Autodesk Inventor part; units mm, degrees
ref_plane "YZ Plane" through (0, 0, 0) normal (1, 0, 0) x (0, 1, 0)
ref_plane "XZ Plane" through (0, 0, 0) normal (0, 1, 0) x (-1, 0, 0)
ref_plane "XY Plane" through (0, 0, 0) normal (0, 0, 1) x (1, 0, 0)
sketch "Sketch1" plane through (0, 0, 0) normal (0, 1, 0) x (-1, 0, 0)
  point P0 (0, 0)
sketch "Sketch2" plane through (0, 0, 0) normal (0, 1, 0) x (-1, 0, 0)
  line L0 (70, -12) -> (70, -66)
  line L1 (70, -66) -> (2, -66)
  line L2 (70, -12) -> (2, -12)
  line L3 (2, -66) -> (2, -12)
  point P0 (0, 0)
  point P1 (2, 0)
  dimension "d151" = 68
  dimension "d152" = 54
extrude "Extrusion1" add sketch "Sketch2" along normal blind 14
sketch "Sketch3" plane through (0, 14, 0) normal (0, 1, 0) x (1, 0, 0)
  point P0 (0, 0)
sketch "Sketch4" plane through (0, 14, 0) normal (0, 1, 0) x (1, 0, 0)
  line L0 (-2, 66) -> (-70, 66)
  line L1 (-30.4814, 66) -> (-28.4814, 66)
  line L2 (-28.4814, 66) -> (-28.4814, 64)
  line L3 (-70, 66) -> (-70, 12)
  line L4 (-70, 37.8423) -> (-70, 39.8423)
  line L5 (-70, 39.8423) -> (-68, 39.8423)
  line L6 (-68, 64) -> (-68, 14)
  line L7 (-68, 64) -> (-4, 64)
  line L8 (-68, 14) -> (-4, 14)
  line L9 (-4, 14) -> (-4, 64)
  line L10 (-70, 12) -> (-2, 12)
  line L11 (-2, 12) -> (-2, 66)
  point P0 (-2, 64)
  point P1 (-68, 12)
  dimension "d6" = 2
  dimension "d8" = 2
  dimension "d102" = 2
  dimension "d104" = 2
  dimension "d153" = 2
  dimension "d154" = 2
extrude "Extrusion2" cut sketch "Sketch4" against normal blind 12 contours L7 L9 L8 L6
sketch "Sketch10" plane through (0, 2, 0) normal (0, 1, 0) x (1, 0, 0)
  line L0 (-48, 14) -> (-48, 17)
  line L1 (-48, 14) -> (-63, 14)
  line L2 (-63, 14) -> (-63, 17)
  line L3 (-63, 17) -> (-48, 17)
  line L4 (-48, 17) -> (-48, 14)
  line L5 (-22, 64) -> (-7, 64)
  line L6 (-7, 64) -> (-7, 61)
  line L7 (-7, 61) -> (-22, 61)
  line L8 (-22, 61) -> (-22, 64)
  line L9 (-68, 64) -> (-4, 64)
  line L10 (-63, 14) -> (-48, 14)
  line L11 (-4, 14) -> (-68, 14)
  point P0 (-68, 2)
  point P1 (-2, 64)
  dimension "d55" = 3
  dimension "d56" = 15
  dimension "d60" = 15
  dimension "d108" = 3
  dimension "d155" = 0
extrude "Extrusion5" add sketch "Sketch10" along normal blind 6
sketch "Sketch12" plane through (0, 0, 0) normal (0, -1, 0) x (1, 0, 0)
  line L0 (0, 0) -> (0, -66)
  line L1 (-2, -12) -> (-2, -66)
  line L2 (-2, -66) -> (-70, -66)
  line L3 (-2, -66) -> (-70, -66)
  line L4 (-36, -66) -> (-36, -12)
  line L5 (-70, -66) -> (-70, -12)
  line L6 (-70, -66) -> (-70, -12)
  line L7 (-70, -39) -> (-2, -39)
  line L8 (-36, -39) -> (-36, -66)
  line L9 (-70, -66) -> (-36, -66)
  arc A0 (-56.4641, -41) -> (-56.4641, -37) centre (-53, -39) ccw
  line L10 (-53, -39) -> (-59.5, -39)
  arc A1 (-59.5, -37) -> (-59.5, -41) centre (-59.5, -39) ccw
  line L11 (-59.5, -41) -> (-56.4641, -41)
  line L12 (-59.5, -37) -> (-56.4641, -37)
  dimension "d158" = 8
  dimension "d159" = 6.5
  dimension "d160" = 4
extrude "Extrusion7" cut sketch "Sketch12" against normal blind 6 contours A0 L11 A1 L7 | L7 A1 L12 A0
sketch "Sketch13" plane through (0, 14, 0) normal (0, 1, 0) x (1, 0, 0)
  line L0 (-70, 66) -> (-70, 12)
  line L1 (-69, 65) -> (-69, 13)
  line L2 (-2, 66) -> (-70, 66)
  line L3 (-68, 64) -> (-4, 64)
  line L4 (-2, 64) -> (-2, 12)
  line L5 (-68, 14) -> (-68, 64)
  line L6 (-4, 14) -> (-68, 14)
  line L7 (-68, 14) -> (-4, 14)
  line L8 (-7, 64) -> (-4, 64)
  line L9 (-4, 14) -> (-4, 64)
  line L10 (-70, 12) -> (-2, 12)
  line L11 (-68, 13) -> (-69, 13)
  line L12 (-68, 13) -> (-3, 13)
  line L13 (-2, 12) -> (-2, 66)
  line L14 (-4, 13) -> (-3, 13)
  line L15 (-3, 13) -> (-3, 64)
  line L16 (-3, 64) -> (-3, 65)
  line L17 (-3, 65) -> (-69, 65)
  dimension "d96" = 1
  dimension "d99" = 1
extrude "Extrusion8" cut sketch "Sketch13" against normal blind 2 contours L17 L16 L15 L12 L11 L1 | L3 L9 L6 L5
sketch "Sketch15" plane through (-70, 0, -66) normal (-1, 0, 0) x (0, 0, 1)
  line L0 (62.4242, 8) -> (52.7396, 8)
  line L1 (0, 0) -> (66, 0)
  line L2 (0, 14) -> (54, 14)
  line L3 (0, 0) -> (0, 14)
  line L4 (18.77, 12) -> (27.77, 12)
  line L5 (27.77, 12) -> (27.77, 17)
  line L6 (27.77, 17) -> (18.77, 17)
  line L7 (18.77, 17) -> (18.77, 12)
  point P0 (66, 14)
  dimension "d118" = 8
  dimension "d140" = 27.77
  dimension "d141" = 9
  dimension "d143" = 5
  dimension "d150" = 4
extrude "Extrusion9" cut sketch "Sketch15" against normal blind 10
sketch "Sketch16" plane through (-2, 0, -66) normal (0, 0, -1) x (-1, 0, 0)
  line L0 (39.4, 14) -> (47.9, 14)
  line L1 (47.9, 14) -> (47.9, 9)
  line L2 (47.9, 9) -> (39.4, 9)
  line L3 (39.4, 9) -> (39.4, 14)
  line L4 (54.5, 14) -> (63, 14)
  line L5 (63, 14) -> (63, 9)
  line L6 (63, 9) -> (54.5, 9)
  line L7 (54.5, 9) -> (54.5, 14)
  line L8 (20, 8) -> (5, 8)
  line L9 (68, 0) -> (68, 14)
  point P0 (-2, 0)
  dimension "d127" = 8.5
  dimension "d128" = 8.5
  dimension "d131" = 28.6
  dimension "d132" = 13.5
  dimension "d148" = 5
  dimension "d149" = 6
extrude "Extrusion10" cut sketch "Sketch16" against normal blind 10
fillet "Fillet8" radius 3 1 edges at (-70, 7, -66)
sketch "Sketch17" plane through (0, 2, 0) normal (0, 1, 0) x (1, 0, 0)
  arc A0 (-59.5, 42) -> (-59.5, 36) centre (-59.5, 39) ccw
  line L0 (-59.5, 42) -> (-57, 42)
  arc A1 (-57, 36) -> (-57, 42) centre (-53, 39) ccw
  line L1 (-57, 36) -> (-59.5, 36)
  point P0 (0, 0)
extrude "Extrusion11" add sketch "Sketch17" along normal blind 5
properties part number "Shell 4 bottom"
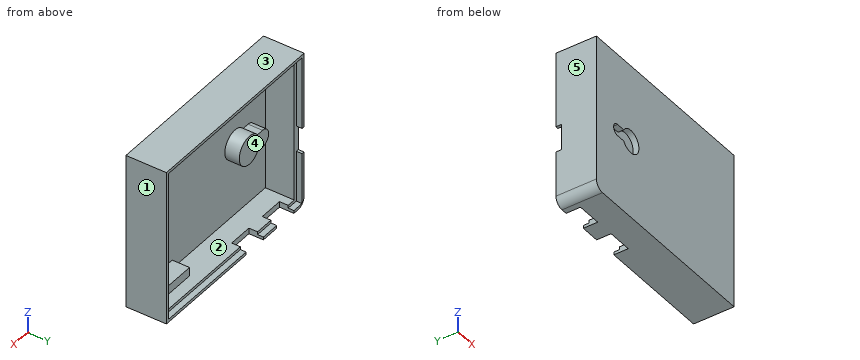
Model file for the job. Use its own axes, mm. Face numbers are marked on the shaded views. A direction names the side the tool comes from. Give positions to 0.01 mm unless a question says otherwise; leave off trailing zeros. Order: outer loops, then holes, each group sorted by start corner. A loop starts at its lowest first (then second) coordinate and runs counter-clockwise, first axis right, second up. Notation, with made-up numbers: (-29, 7.25) - (-23, 7.25) arc R32 cw to (-23, 43.25) - close; hole circle Ø1 at (20, 80.5). An arc over 180 degrees is marked (long way). Write item = value, one per line. Start each with the question number.
1. Cut at B-B, the plane z = -57.5. List the corners of the cut face in (x, y).
2. Probe line 1 along Z through (x, y) = (-18.5, 7.75); line 2 along X through (y, z) = (1.5, -39); line 3 along Z through (x, y) = (-41, 8.25). List the from-to ranges inside material, lowest first.
3. Drop flat-ended pins along their axis: P1, Ø3, axis at x = -62.5, z = -47, coming from the +Y side; P2, Ø2, axis at y = 11.5, z = -65, coming from the -X side. Give the stop position or say it passes through.
4. Cut at C-C, the plane x = -37. List the corners of the cut face in (y, z).
5. Cut at A-A, the plane y = 5.5. List the corners of the cut face in (x, z).
6. Two-plate mould, pull along Z, no slides. Class the marked faces 1, 2 and 3: pulls with the +Z half, pulls with the -Z half, needs draft (parallel to the pull), parting line crosses it, or undercut.
7. Which spindle directions (+Z, -Z, +X, -X, +Y, -Y) get a long thin tool onto all of the face, cutting with end or side? Do the marked faces 4 and 5. Say none if no direction does.
8. Cut at D-D, the plane x = -53. List the corners of the cut face in (y, z), and give its area (3 significant figures).
Taken from the geometry:
q1.outline = (-70, 0) - (-2, 0) - (-2, 14) - (-3, 14) - (-3, 12) - (-4, 12) - (-4, 2) - (-68, 2) - (-68, 12) - (-69, 12) - (-69, 14) - (-70, 14) - close
q2.line_1 = -66 to -61, -14 to -12
q2.line_2 = -70 to -61.5, -49 to -2
q2.line_3 = -66 to -64, -14 to -12
q3.P1 = 2
q3.P2 = -69.83
q4.outline = (0, -66) - (14, -66) - (14, -65) - (12, -65) - (12, -64) - (2, -64) - (2, -14) - (12, -14) - (12, -13) - (14, -13) - (14, -12) - (0, -12) - close
q5.outline = (-70, -63) arc R3 ccw to (-67, -66) - (-2, -66) - (-2, -12) - (-70, -12) - close; (-59.5, -42) - (-57, -42) arc R5 ccw (long way) to (-57, -36) - (-59.5, -36) arc R3 ccw to start; hole (-68, -64) - (-22, -64) - (-22, -61) - (-7, -61) - (-7, -64) - (-4, -64) - (-4, -14) - (-48, -14) - (-48, -17) - (-63, -17) - (-63, -14) - (-68, -14) - close
q6.face_1 = needs draft
q6.face_2 = undercut
q6.face_3 = pulls with the +Z half
q7.face_4 = +Y
q7.face_5 = +Z, -Z, -X, +Y, -Y
q8.outline = (0, -66) - (14, -66) - (14, -65) - (12, -65) - (12, -64) - (2, -64) - (2, -44) - (7, -44) - (7, -34) - (2, -34) - (2, -17) - (8, -17) - (8, -14) - (12, -14) - (12, -13) - (14, -13) - (14, -12) - (0, -12) - (0, -35) - (2, -35) - (2, -43) - (0, -43) - close
q8.area = 204 mm²
